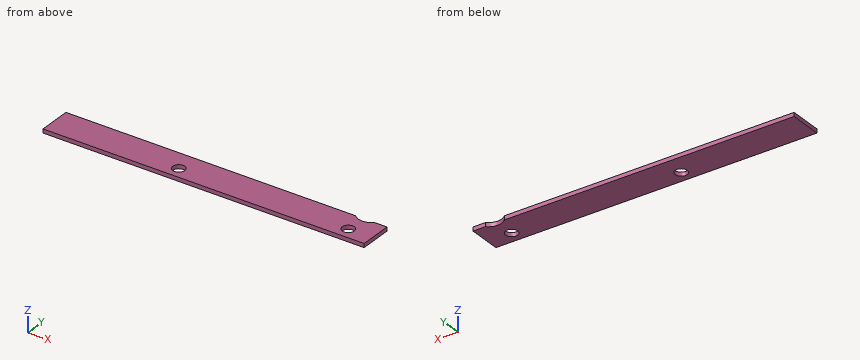
```python
from build123d import *

# Parameters (mm, degrees)
SALIENTE_EXTRUIR1_DEPTH = 12
CROQUIS2_R              = 18.5
CORTAR_EXTRUIR1_DEPTH   = 13
CROQUIS3_R              = 18.5
CORTAR_EXTRUIR2_DEPTH   = 13


with BuildPart() as part:
    # Croquis1 → Saliente-Extruir1 (new body)
    with BuildSketch(Plane.XY):
        with BuildLine():
            Line((0, 0), (985, 0))
            Line((985, 0), (985, 100))
            Line((985, 100), (946.952353927, 100))
            ThreePointArc((946.952353927, 100), (918, 88.021483703), (889.047646073, 100))
            Line((889.047646073, 100), (0, 100))
            Line((0, 100), (0, 0))
        make_face()
    extrude(amount=SALIENTE_EXTRUIR1_DEPTH)

    # Croquis2 → Cortar-Extruir1 (cut, through all)
    with BuildSketch(Plane.XY.offset(12)):
        with Locations((911, 36.5)):
            Circle(CROQUIS2_R)
    extrude(amount=-CORTAR_EXTRUIR1_DEPTH, mode=Mode.SUBTRACT)

    # Croquis3 → Cortar-Extruir2 (cut, through all)
    with BuildSketch(Plane.XY.offset(12)):
        with Locations((391, 36.5)):
            Circle(CROQUIS3_R)
    extrude(amount=-CORTAR_EXTRUIR2_DEPTH, mode=Mode.SUBTRACT)


solid = part.part
```
Build history of the part. All positions in model axes, mm. Coordinates: 2 decimals unless noted, no trailing zeros. Order: outer loops, then holes, each group sorted by start corner. A loop starts at its lowest first (then second) coordinate and runs counter-clockwise, first axis right, second up.
Item 1: Saw through at D-D on x = 911. List the corners of the cut face in (y, z).
Filled in:
outline: (0, 0) - (18, 0) - (18, 12) - (0, 12) - close; (55, 0) - (88.62, 0) - (88.62, 12) - (55, 12) - close
Item 2: Saw through at C-C on y = 36.5. List the corners of the cut face in (x, z).
Filled in:
outline: (0, 0) - (372.5, 0) - (372.5, 12) - (0, 12) - close; (409.5, 0) - (892.5, 0) - (892.5, 12) - (409.5, 12) - close; (929.5, 0) - (985, 0) - (985, 12) - (929.5, 12) - close
Item 3: Drill centre lines: L1, parallel to X at y = 34, z = 3.5; L2, parallel to X at y = 35, z = 8.75; L3, parallel to Y at x = 911, z = 5.5. Where is each one in solid material? Low to high.
Filled in:
L1: x = 0 to 372.67, 409.33 to 892.67, 929.33 to 985
L2: x = 0 to 372.56, 409.44 to 892.56, 929.44 to 985
L3: y = 0 to 18, 55 to 88.62
Item 4: Saw through at B-B on x = 391. List the corners of the cut face in (y, z), then the cut area to 3 significant figures.
Filled in:
outline: (0, 0) - (18, 0) - (18, 12) - (0, 12) - close; (55, 0) - (100, 0) - (100, 12) - (55, 12) - close
area: 756 mm2
Item 5: Saw through at A-A on z = 9.5. List the corners of the cut face in (x, y).
Filled in:
outline: (0, 0) - (985, 0) - (985, 100) - (946.95, 100) arc R40.98 cw to (889.05, 100) - (0, 100) - close; hole circle Ø37 at (391, 36.5); hole circle Ø37 at (911, 36.5)
